Autodesk Inventor part; units mm, degrees
ref_plane "Work Plane1" through (0, -10, 0) normal (0, 0, -1) x (0, 1, 0)
ref_plane "Work Plane3" through (0, 0, 1.9812) normal (-1, 0, 0) x (0, 1, 0)
ref_plane "YZ Plane" through (0, 0, 0) normal (1, 0, 0) x (0, 1, 0)
sketch "Esquisse1" plane through (0, 0, 0) normal (0, 1, 0) x (-1, 0, 0)
  arc A0 (-2.9084, 3.4932) -> (-2.9084, -3.4932) centre (-4.7244, 0) ccw
  arc A1 (-3.9147, 1.7803) -> (-3.9147, -1.7803) centre (-4.7244, 0) ccw
  line L0 (0, 1.9812) -> (60.96, 1.9812)
  line L1 (0, -1.9812) -> (60.96, -1.9812)
  line L2 (60.96, 1.9812) -> (76.2, 7.8199)
  line L3 (76.2, 7.8199) -> (76.8619, 6.0923)
  line L4 (76.8619, 6.0923) -> (60.96, 0)
  line L5 (60.96, 0) -> (78.6399, -6.7735)
  line L6 (78.6399, -6.7735) -> (77.978, -8.5011)
  line L7 (77.978, -8.5011) -> (60.96, -1.9812)
  line L8 (0, 0) -> (-3.9147, -1.7803)
  line L9 (0, 0) -> (-3.9147, 1.7803)
  line L10 (0, 1.9812) -> (0, -1.9812) construction
  line L11 (0, 1.9812) -> (-2.9084, 3.4932)
  line L12 (0, -1.9812) -> (-2.9084, -3.4932)
  line L13 (-8.6614, 0) -> (60.96, 0) construction
  line L14 (60.96, 1.9812) -> (60.96, -1.9812) construction
  dimension "d0" = 60.96
  dimension "d1" = 76.2
  dimension "d2" = 159.037
  dimension "d3" = 159.037
  dimension "d4" = 1.778
  dimension "d5" = 1.9558
  dimension "d6" = 3.937
  dimension "d7" = 1.9812
  dimension "d8" = 1.9812
  dimension "d9" = 4.7244
extrude "Corps" add sketch "Esquisse1" along normal mid plane 3.9624
fillet "Congé" radius 1.3868 14 edges at (-68.58, -1.9812, 4.9006) (-68.58, 1.9812, 4.9006) (-30.48, -1.9812, 1.9812) (-30.48, 1.9812, 1.9812) (8.6614, -1.9812, 0) (1.4542, -1.9812, -2.7372) (1.4542, -1.9812, 2.7372) (8.6614, 1.9812, 0) (1.4542, 1.9812, 2.7372) (1.4542, 1.9812, -2.7372) (-30.48, -1.9812, -1.9812) (-69.469, -1.9812, -5.2412) (-30.48, 1.9812, -1.9812) (-69.469, 1.9812, -5.2412)
ref_plane "Work Plane1" through (0, -10, 0) normal (0, 0, -1) x (0, 1, 0)
ref_plane "Work Plane3" through (0, 0, 1.9812) normal (-1, 0, 0) x (0, 1, 0)
equation "\"d0\" = MSIAB"
equation "\"d1\" = SNLG"
equation "\"d4\" = LGDIF"
equation "\"d5\" = -0.5 * SNND1 + 0.5 * KBR"
equation "\"d6\" = 0.5 * KBR"
equation "\"d7\" = 0.5 * SNND1"
equation "\"d8\" = 0.5 * SNND1"
equation "\"d9\" = KOL - 0.5 * KBR"
equation "\"d10\" = SNND1"
equation "\"d12\" = 0.35 * SNND1"
equation "\"SNND\" = 3.96875"
equation "\"SNLG\" = 76.2"
equation "\"SNND1\" = 3.9624"
equation "\"KBR\" = 7.874"
equation "\"KOL\" = 8.6614"
equation "\"LGDIF\" = 1.778"
equation "\"MSIAB\" = 60.96"
equation "\"NNDMAX\" = 22.225"
equation "\"DSH\" = 5.953"
equation "\"NNDMIN\" = 15.875"
equation "\"SPBOR\" = 4.3688"
properties part number "SAE J487a - 5/32 x 3   Type fourche" material "Acier doux"
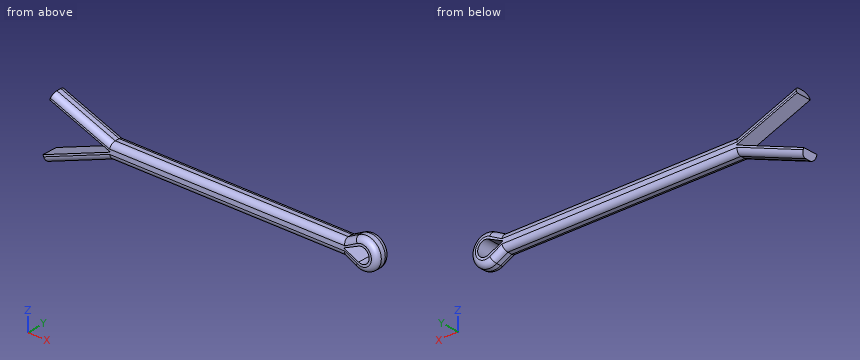
Read the model definition and answer for the solid it produces. Units are mm, in the model's axes. Give positions to 0.01 mm unless a question says otherwise; leave off trailing zeros. Write each loop counter-clockwise with the first axis right and the second up, starting at its lowest first coordinate (ties: lowest second). Pieces come first, ordered by that corner, then holes. Notation, with made-up numbers: M 69,12 L 79,12 A17 ccw 79,28 Z; hole C -24,42.5 d9. An arc over 180 degrees is marked long. Put each result on its own line as item: value. Start each with the question number.
1. The part is cut by section A-A, the plane x = -26. Give the vertices of the cut face in (y, z).
2. The part is cut by section B-B, the plane y = 1.2. Give the vertices of the cut face in (x, z).
3. Each of these flat-tipped pins is pushed along its axis until it touches: pin 1 Ø1 at (x, y) = (-33, 0) entering from -Z; pin 2 Ø2 at (x, z) = (-69, -1.5) entering from +Y. Where does it stop, or does it pass through?
4. Consider line 1 along Z through (x, y) = (-4, -0.1); line 2 along Z through (x, y) = (1.5, 1.7); line 3 along Z through (x, y) = (2, 0). Determine where each line is inside the solid, lowest interval first.
Final values:
1. outline: M -1.98,-0.59 A1.39 ccw -0.59,-1.98 L 0.59,-1.98 A1.39 ccw 1.98,-0.59 L 1.98,0.59 A1.39 ccw 0.59,1.98 L -0.59,1.98 A1.39 ccw -1.98,0.59 Z
2. outline: M -78.64,-6.77 L -78.03,-8.37 L -60.99,-1.84 L 0.03,-1.84 L 2.97,-3.37 A3.8 ccw long 2.97,3.37 L 0.03,1.84 L -60.99,1.84 L -76.25,7.69 L -76.86,6.09 L -60.96,0 Z; hole M 0,0 L 3.91,-1.78 A1.96 ccw long 3.91,1.78 Z
3. pin 1: stops at z = -1.98
3. pin 2: passes through
4. line 1: z = -1.98 to 1.98
4. line 2: z = -2.14 to -0.68, 0.68 to 2.14
4. line 3: z = -3.02 to -0.91, 0.91 to 3.02
